Geometry: final body of the model. Coordinates: model frame, mm. Face numbers are marked on the shaded views. A direction names the side the tool comes from. Give positions to 0.01 mm unless a question says otherwise; leave off trailing zeros. Loops run counter-clockwise (first coordinate to the right, second up) from the corner with the lowest first, then second, coordinate; pieces in that order, holes last. Notation, with made-up numbers: (-37, 21.25) -> (-25, 21.25) arc R18 ccw to (-25, 42.25) -> close; hole circle Ø5 at (-33.75, -4). An arc over 180 degrees is marked (long way). One line per question, with ' | ' between items. Start each with the question number.
Item 1: Section B-B on z = 31. Return loops of the section in (x, y), then the cut area to 3 significant figures.
Item 2: Set-up query: the marked faces 1 and 2. Return all of +Z, -Z, +X, -X, +Y, -Y with unobstructed straight access to the full face (end or side cutting, diameter ignored); none if empty.
Item 3: Section C-C on x = 10. Return loops of the section in (y, z), then the cut area to 3 significant figures.
Item 4: Section A-A on y = 0. Return loops of the section in (x, z), then the cut area to 3 significant figures.
Item 5: Pin query (flat end, axial travel): P1, Ø2, axis at x = 66, y = -14.5, coming from the -Z side; P2, Ø8, axis at x = 83.5, y = -13, coming from the -Z side; P3, Ø2, axis at x = 66.5, y = 19, coming from the -Z side; P4, Ø8, axis at y = 2.5, z = -22, coming from the -X side. Return the tip coordinate at first contact, or that it passes through.
Item 6: Material intervals for line 1 along Z through (x, y) = (39, 0); line 2 along X through (y, z) = (32, 5); line 3 along Y through (x, z) = (36.5, 7.5), sorted ascending. Write a range as [from, to].
Item 7: Mould query, pull axis Y, two halves, no side actions, for the marked faces 3, 4, 5 and 6. Classes: released by +Y, released by -Y, zero draft, split by the parting line, or undercut.
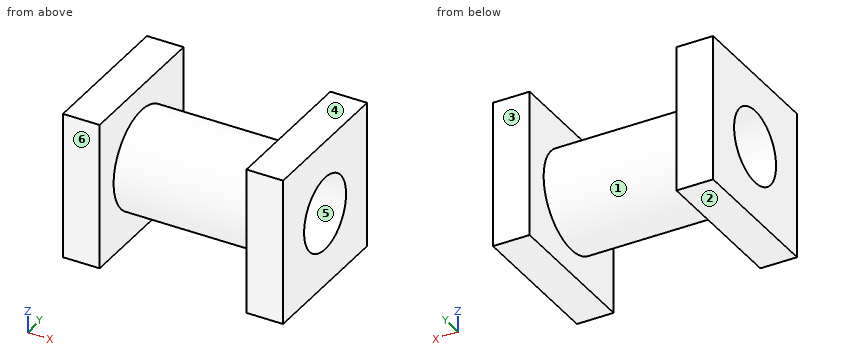
from build123d import *

# Parameters (mm, degrees)
F0_W     = 76.2
F0_H     = 76.2
F1_DEPTH = 19.05
F2_R     = 25.4
F3_DEPTH = 76.2
F4_W     = 76.2
F4_H     = 76.2
F4_R     = 25.4
F5_DEPTH = 19.05
F6_R     = 19.05
F7_DEPTH = 114.3


with BuildPart() as f1:
    # F0 (on Right) → F1 (new body)
    with BuildSketch(Plane.YZ):
        Rectangle(F0_W, F0_H)
    extrude(amount=F1_DEPTH)

    # F2 (on face) → F3 (join)
    with BuildSketch(Plane.YZ.offset(19.05)):
        Circle(F2_R)
    extrude(amount=F3_DEPTH)

    # F4 (on face) → F5 (join)
    with BuildSketch(Plane.YZ.offset(95.25)):
        Rectangle(F4_W, F4_H)
        Circle(F4_R, mode=Mode.SUBTRACT)
        Circle(F4_R)
    extrude(amount=F5_DEPTH)

    # F6 (on face) → F7 (cut)
    with BuildSketch(Plane(origin=(0, 0, 0), x_dir=(0, -1, 0), z_dir=(-1, 0, 0))):
        Circle(F6_R)
    extrude(amount=-F7_DEPTH, mode=Mode.SUBTRACT)


solid = f1.part
Result sheet:
1) outline: (0, -38.1) -> (19.05, -38.1) -> (19.05, 38.1) -> (0, 38.1) -> close; (95.25, -38.1) -> (114.3, -38.1) -> (114.3, 38.1) -> (95.25, 38.1) -> close | area: 2,900 mm²
2) face 1: none | face 2: -Z, +X, -X, +Y, -Y
3) outline: (-38.1, -38.1) -> (38.1, -38.1) -> (38.1, 38.1) -> (-38.1, 38.1) -> close; hole circle Ø38.1 at (0, 0) | area: 4,670 mm²
4) outline: (0, -38.1) -> (19.05, -38.1) -> (19.05, -25.4) -> (95.25, -25.4) -> (95.25, -38.1) -> (114.3, -38.1) -> (114.3, -19.05) -> (0, -19.05) -> close; (0, 19.05) -> (114.3, 19.05) -> (114.3, 38.1) -> (95.25, 38.1) -> (95.25, 25.4) -> (19.05, 25.4) -> (19.05, 38.1) -> (0, 38.1) -> close | area: 2,420 mm²
5) P1: stops at z = -21.52 | P2: stops at z = -23.75 | P3: stops at z = -17.92 | P4: stops at x = 0
6) line 1: z = [-25.4, -19.05], [19.05, 25.4] | line 2: x = [0, 19.05], [95.25, 114.3] | line 3: y = [-24.27, -17.51], [17.51, 24.27]
7) face 3: released by +Y | face 4: zero draft | face 5: undercut | face 6: released by -Y
